Answer from the drawing. Dimensions are ordinates in mm from the lowest x, y and z of the part. A direction names the side the tool comes from. Round coordinates to 2 decimals unless told otherwise and drop trailing zeros. Write each loop counter-clockwise with the first axis right and the second up, starting at its lowest first coordinate (ties: lowest second). Pieces come first, ordered by that corner, then holes. Notation, with made-up numbers: (41.5, 86) - (82.5, 86) arc R19 ccw to (82.5, 96) - close; hole circle Ø2 at (-2.5, 76.25). An arc over 180 degrees is marked (long way). Answer as a JSON object with one key per item and string values.
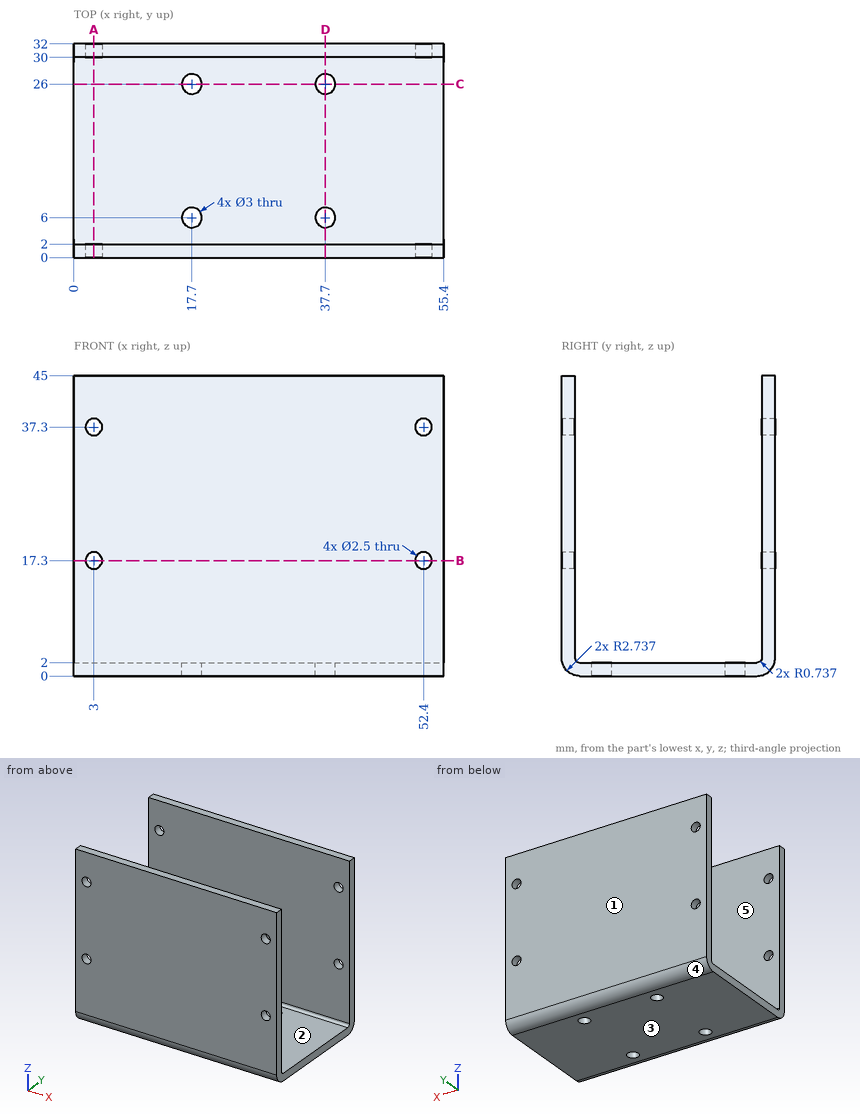
Item 1: A cutting plane is placed at C-C (y = 26). Write down the section's boundary in (x, z).
Results found:
{"outline": "(0, 0) - (16.2, 0) - (16.2, 2) - (0, 2) - close; (19.2, 0) - (36.2, 0) - (36.2, 2) - (19.2, 2) - close; (39.2, 0) - (55.4, 0) - (55.4, 2) - (39.2, 2) - close"}
Item 2: Consider line 1 along X through (y, z) = (1.2, 17.3); line 2 along Y through (x, z) = (52.5, 34); line 3 along Z through (x, y) = (52, 1) (1 decimal). Determine where each line is inside the solid, lowest interval first.
Results found:
{"line 1": "0 to 1.75, 4.25 to 51.15, 53.65 to 55.4", "line 2": "0 to 2, 30 to 32", "line 3": "0.6 to 16.1, 18.5 to 36.1, 38.5 to 45"}
Item 3: A cutting plane is placed at D-D (x = 37.7). Write down the section's boundary in (y, z).
Results found:
{"outline": "(0, 2.74) arc R2.74 ccw to (2.74, 0) - (4.5, 0) - (4.5, 2) - (2.74, 2) arc R0.74 cw to (2, 2.74) - (2, 45) - (0, 45) - close; (7.5, 0) - (24.5, 0) - (24.5, 2) - (7.5, 2) - close; (27.5, 0) - (29.26, 0) arc R2.74 ccw to (32, 2.74) - (32, 45) - (30, 45) - (30, 2.74) arc R0.74 cw to (29.26, 2) - (27.5, 2) - close"}
Item 4: Determine the mould class of the marked faces 3, 4 and 5 for opening direction Y: pulls with the +Y half, pulls with the -Y half, needs draft (parallel to the pull), parting line crosses it, or undercut.
Results found:
{"face 3": "needs draft", "face 4": "pulls with the +Y half", "face 5": "undercut"}
Item 5: A cutting plane is placed at B-B (z = 17.3). Write down the section's boundary in (x, y).
Results found:
{"outline": "(0, 0) - (1.75, 0) - (1.75, 2) - (0, 2) - close; (0, 30) - (1.75, 30) - (1.75, 32) - (0, 32) - close; (4.25, 0) - (51.15, 0) - (51.15, 2) - (4.25, 2) - close; (4.25, 30) - (51.15, 30) - (51.15, 32) - (4.25, 32) - close; (53.65, 0) - (55.4, 0) - (55.4, 2) - (53.65, 2) - close; (53.65, 30) - (55.4, 30) - (55.4, 32) - (53.65, 32) - close"}
Item 6: For the marked faces 1 and 2, determine the directions among +Z, -Z, +X, -X, +Y, -Y from which every point of the face is accessible in a straight line to the end or side of a thin tool.
Results found:
{"face 1": "+Z, -Z, +X, -X, +Y", "face 2": "+Z, +X, -X"}
Item 7: A cutting plane is placed at A-A (x = 3). Write down the section's boundary in (y, z).
Results found:
{"outline": "(0, 2.74) arc R2.74 ccw to (2.74, 0) - (29.26, 0) arc R2.74 ccw to (32, 2.74) - (32, 16.05) - (30, 16.05) - (30, 2.74) arc R0.74 cw to (29.26, 2) - (2.74, 2) arc R0.74 cw to (2, 2.74) - (2, 16.05) - (0, 16.05) - close; (0, 18.55) - (2, 18.55) - (2, 36.05) - (0, 36.05) - close; (0, 38.55) - (2, 38.55) - (2, 45) - (0, 45) - close; (30, 18.55) - (32, 18.55) - (32, 36.05) - (30, 36.05) - close; (30, 38.55) - (32, 38.55) - (32, 45) - (30, 45) - close"}
Item 8: This flat-tipped pin is pushed along its axis until it touches: P1, Ø12, axis at x = 21, y = 10, coming from the +Z side. Where does it stop, or does it pass through?
Results found:
{"P1": "z = 2"}
